Could you check a few things on this model? Use its own coordinates, in mm. Face numbers are marked on the shaded views. A direction names the side the tool comes from. Give positions to 0.01 mm unless a question says otherwise; leave off trailing zeros. Loops run counter-clockwise (first coordinate to the right, second up) from the corner with the lowest first, then second, coordinate; pieces in that order, holes last. Notation, with made-up numbers: (85, 57) - (142, 57) arc R28 ccw to (142, 81) - close; hole circle Ø4 at (34, 17). An arc over 180 degrees is marked (long way). Answer in a Markdown table with one row per item. Add a question column.
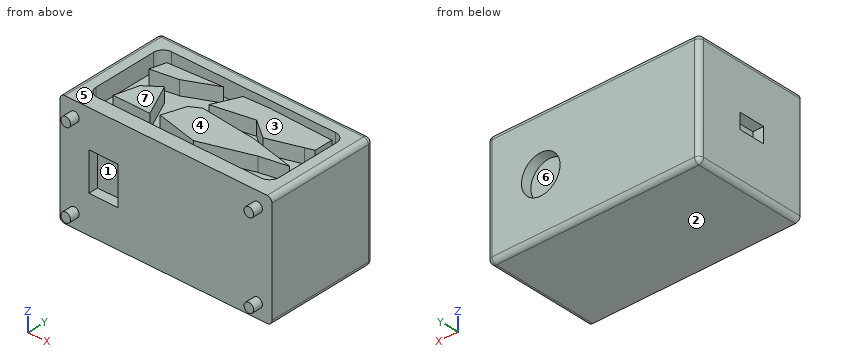
```python
from build123d import *

# Parameters (mm, degrees)
SKETCH1_W           = 220
SKETCH1_H           = 100
SKETCH1_W_2         = 184
SKETCH1_H_2         = 64
BOSS_EXTRUDE1_DEPTH = 80
SKETCH11_W          = 220
SKETCH11_H          = 100
BOSS_EXTRUDE6_DEPTH = 18
SKETCH12_W          = 220
SKETCH12_H          = 100
BOSS_EXTRUDE7_DEPTH = 18
SKETCH2_W           = 220
SKETCH2_H           = 116
SKETCH2_W_2         = 190
SKETCH2_H_2         = 86
BOSS_EXTRUDE2_DEPTH = 18
BOSS_EXTRUDE3_DEPTH = 15
FILLET9_R           = 5
FILLET8_R           = 10
SKETCH13_R          = 5
BOSS_EXTRUDE8_DEPTH = 10
SKETCH14_W          = 16
SKETCH14_H          = 27
CUT_EXTRUDE1_DEPTH  = 10
CUT_EXTRUDE1_DRAFT  = -6
SKETCH15_R          = 20
CUT_EXTRUDE2_DEPTH  = 10
CUT_EXTRUDE2_DRAFT  = -4
SKETCH17_W          = 30
SKETCH17_H          = 40
CUT_EXTRUDE3_DEPTH  = 10


with BuildPart() as part:
    # Sketch1 → Boss-Extrude1 (new body)
    with BuildSketch(Plane(origin=(0, 0, 0), x_dir=(1, 0, 0), z_dir=(0, 1, 0))):
        with Locations((19.985024942, -17.460570406)):
            Rectangle(SKETCH1_W, SKETCH1_H)
        with Locations((19.985024942, -17.460570406)):
            Rectangle(SKETCH1_W_2, SKETCH1_H_2, mode=Mode.SUBTRACT)
    extrude(amount=BOSS_EXTRUDE1_DEPTH)

    # Sketch11 → Boss-Extrude6 (add)
    with BuildSketch(Plane(origin=(0, 80, 0), x_dir=(1, 0, 0), z_dir=(0, 1, 0))):
        with Locations((19.985024942, -17.460570406)):
            Rectangle(SKETCH11_W, SKETCH11_H)
    extrude(amount=BOSS_EXTRUDE6_DEPTH)

    # Sketch12 → Boss-Extrude7 (add)
    with BuildSketch(Plane.XZ):
        with Locations((19.985024942, 17.460570406)):
            Rectangle(SKETCH12_W, SKETCH12_H)
    extrude(amount=BOSS_EXTRUDE7_DEPTH)

    # Sketch2 → Boss-Extrude2 (add)
    with BuildSketch(Plane.XY.offset(67.460570406)):
        with Locations((19.985024942, 40)):
            Rectangle(SKETCH2_W, SKETCH2_H)
        with Locations((19.985024942, 40)):
            Rectangle(SKETCH2_W_2, SKETCH2_H_2, mode=Mode.SUBTRACT)
    extrude(amount=BOSS_EXTRUDE2_DEPTH)

    # Sketch3 → Boss-Extrude3 (add)
    with BuildSketch(Plane.XY.offset(67.460570406)):
        Polygon((14.957915815, 76.501183659), (2.936567903, 50.272788216), (44.902000614, 58.797016735), (65.229007083, 43.497119393), (98.451641312, 54.534902475), (106.944672327, 57.35660028), (106.944672327, 76.501183659), (41.011301547, 77.951227522), align=None)
        Polygon((-60.667291048, 72.566924343), (-65.038690289, 56.611317114), (-37.280305111, 61.419856279), (-5.369090654, 76.501183659), align=None)
        Polygon((-54.547332111, 34.535750949), (-39.247434769, 46.119958937), (-22.636117654, 10.711625088), (-60.667291048, 10.711625088), align=None)
        Polygon((-7.554790274, 37.377160456), (-15.111155502, 14.241854245), (27.984608681, 4.591666151), (79.685296007, 21.768539242), (107.463223985, 27.410930863), (60.959158385, 37.824320409), (2.936567903, 43.497119393), align=None)
    extrude(amount=BOSS_EXTRUDE3_DEPTH)

    # Fillet9
    fillet9_edges = [part.edges().sort_by_distance(p)[0] for p in [
        (-90.014975058, 98, 26.460570406),
        (129.985024942, 98, 26.460570406),
        (19.985024942, 98, -32.539429594),
        (19.985024942, 98, 85.460570406),
        (-90.014975058, 40, 85.460570406),
        (129.985024942, 40, 85.460570406),
        (-90.014975058, 40, -32.539429594),
        (129.985024942, 40, -32.539429594),
    ]]
    fillet(fillet9_edges, radius=FILLET9_R)

    # Fillet8
    fillet8_edges = [part.edges().sort_by_distance(p)[0] for p in [
        (-75.014975058, 83, 76.460570406),
        (114.985024942, 83, 76.460570406),
        (114.985024942, -3, 76.460570406),
        (-75.014975058, -3, 76.460570406),
    ]]
    fillet(fillet8_edges, radius=FILLET8_R)

    # Sketch13 → Boss-Extrude8 (add)
    with BuildSketch(Plane.XZ.offset(18)):
        with Locations(Location((-75.014975058, 70.460570406, 0), (0, 0, 270))):
            Circle(SKETCH13_R)
        with Locations(Location((114.985024942, 70.460570406, 0), (0, 0, 90))):
            Circle(SKETCH13_R)
        with Locations(Location((114.985024942, -17.539429594, 0), (0, 0, 270))):
            Circle(SKETCH13_R)
        with Locations(Location((-75.014975058, -17.539429594, 0), (0, 0, 90))):
            Circle(SKETCH13_R)
    extrude(amount=BOSS_EXTRUDE8_DEPTH)


with BuildPart() as cut_extrude1_tool:
    # Sketch14 → Cut-Extrude1 (with draft: the straight prism first)
    with BuildSketch(Plane.ZY.offset(90.014975058)):
        with Locations((26.460570406, 37.5)):
            Rectangle(SKETCH14_W, SKETCH14_H)
    extrude(amount=-CUT_EXTRUDE1_DEPTH)
    # Cut-Extrude1: the draft: its side faces are tilted about the plane it starts from
    cut_extrude1_sides = [cut_extrude1_tool.faces().sort_by_distance(p)[0] for p in [
        (-85.014975058, 37.5, 18.460570406),
        (-85.014975058, 24, 26.460570406),
        (-85.014975058, 37.5, 34.460570406),
        (-85.014975058, 51, 26.460570406),
    ]]
    draft(cut_extrude1_sides, Plane.ZY.offset(90.014975058), CUT_EXTRUDE1_DRAFT)


with BuildPart() as part_1:
    add(part.part)

    # Cut-Extrude1: cut by cut_extrude1_tool
    add(cut_extrude1_tool.part, mode=Mode.SUBTRACT)


with BuildPart() as cut_extrude2_tool:
    # Sketch15 → Cut-Extrude2 (with draft: the straight prism first)
    with BuildSketch(Plane(origin=(0, 98, 0), x_dir=(1, 0, 0), z_dir=(0, 1, 0))):
        with Locations((74.457875253, -26.460570406)):
            Circle(SKETCH15_R)
    extrude(amount=-CUT_EXTRUDE2_DEPTH)
    # Cut-Extrude2: the draft: its side faces are tilted about the plane it starts from
    cut_extrude2_sides = [cut_extrude2_tool.faces().sort_by_distance(p)[0] for p in [
        (54.457875253, 93, 26.460570406),
    ]]
    draft(cut_extrude2_sides, Plane(origin=(0, 98, 0), x_dir=(1, 0, 0), z_dir=(0, 1, 0)), CUT_EXTRUDE2_DRAFT)


with BuildPart() as part_2:
    add(part_1.part)

    # Cut-Extrude2: cut by cut_extrude2_tool
    add(cut_extrude2_tool.part, mode=Mode.SUBTRACT)

    # Sketch17 → Cut-Extrude3 (cut)
    with BuildSketch(Plane.XZ.offset(18)):
        with Locations((-45.014975058, 26.460570406)):
            Rectangle(SKETCH17_W, SKETCH17_H)
    extrude(amount=-CUT_EXTRUDE3_DEPTH, mode=Mode.SUBTRACT)


solid = part_2.part
```
(1) I want a section at A-A on z = -5. Please give me the cut outline in (x, y).
(2) On a 3-axis mill with a long thin cutter (end or side, diameter ignored), from which of +Z, -Z, +X, -X, +Y, -Y can I reach the whole of each face in a straight line? I mean the marked faces 1, 2 and 3. Say none if no direction works.
(3) We'd pull the mould along Y, two halves only. Please class the marked faces 4, 5, 6 and 7: pulls with the +Y half, pulls with the -Y half, needs draft (parallel to the pull), parting line crosses it, or undercut.
(4) I want a section at D-D on y = 65.5. Please give me the cut outline in (x, z), then the cut area to 3 significant figures.
(5) For pin 1 Ø1 at (x, z) = (-28.5, 40.5) entering from -Y; pin 2 Ø10 at (x, y) = (81.5, 19) entering from +Z; pin 3 Ø10 at (x, z) = (-43.5, 23) entering from -Y, each with a flat end and sliding along its axis, tell me the tip position at first contact or that it passes through.
(6) I want a section at B-B on x = -25.5. Please give me the cut outline in (y, z), then the cut area to 3 significant figures.
(7) I want a section at C-C on y = 32. Please give me the cut outline in (x, z).
(8) Please list where these lines run through material, in increasing order: line 1 (Z direction, x = 102.5, y = 31); line 2 (X direction, y = 58.5, z = 17); line 3 (Y direction, x = 85, z = 68.5).
Reported:
| question | item | result |
|---|---|---|
| 1 | outline | (-90.01, -18) - (129.99, -18) - (129.99, 93) arc R5 ccw to (124.99, 98) - (-85.01, 98) arc R5 ccw to (-90.01, 93) - close; hole (-72.01, 0) - (111.99, 0) - (111.99, 80) - (-72.01, 80) - close |
| 2 | face 1 | -Y |
| 2 | face 2 | -Z, +X, -X, +Y, -Y |
| 2 | face 3 | +Z |
| 3 | face 4 | undercut |
| 3 | face 5 | needs draft |
| 3 | face 6 | pulls with the +Y half |
| 3 | face 7 | undercut |
| 4 | outline | (-90.01, -27.54) arc R5 ccw to (-85.01, -32.54) - (124.99, -32.54) arc R5 ccw to (129.99, -27.54) - (129.99, 80.46) arc R5 ccw to (124.99, 85.46) - (114.99, 85.46) - (114.99, 67.46) - (106.94, 67.46) - (106.94, 82.46) - (9.92, 82.46) - (9.92, 67.46) - (-28.65, 67.46) - (-28.65, 82.46) - (-62.6, 82.46) - (-62.6, 67.46) - (-75.01, 67.46) - (-75.01, 85.46) - (-85.01, 85.46) arc R5 ccw to (-90.01, 80.46) - close; hole (-72.01, -14.54) - (111.99, -14.54) - (111.99, 49.46) - (-72.01, 49.46) - close |
| 4 | area | 12,700 mm² |
| 5 | pin 1 | y = -18 |
| 5 | pin 2 | z = 82.46 |
| 5 | pin 3 | y = -8 |
| 6 | outline | (-18, -32.54) - (93, -32.54) arc R5 ccw to (98, -27.54) - (98, 80.46) arc R5 ccw to (93, 85.46) - (83, 85.46) - (83, 67.46) - (75.07, 67.46) - (75.07, 82.46) - (66.99, 82.46) - (66.99, 67.46) - (16.82, 67.46) - (16.82, 82.46) - (10.71, 82.46) - (10.71, 67.46) - (-3, 67.46) - (-3, 85.46) - (-18, 85.46) - close; hole (0, -14.54) - (80, -14.54) - (80, 49.46) - (0, 49.46) - close |
| 6 | area | 7,220 mm² |
| 7 | outline | (-90.01, -27.54) arc R5 ccw to (-85.01, -32.54) - (124.99, -32.54) arc R5 ccw to (129.99, -27.54) - (129.99, 80.46) arc R5 ccw to (124.99, 85.46) - (114.99, 85.46) - (114.99, 67.46) - (86.97, 67.46) - (86.97, 82.46) - (-9.31, 82.46) - (-9.31, 67.46) - (-32.62, 67.46) - (-32.62, 82.46) - (-55.2, 82.46) - (-55.2, 67.46) - (-75.01, 67.46) - (-75.01, 85.46) - (-85.01, 85.46) arc R5 ccw to (-90.01, 80.46) - (-90.01, 34.46) - (-80.01, 33.41) - (-80.01, 19.51) - (-90.01, 18.46) - close; hole (-72.01, -14.54) - (111.99, -14.54) - (111.99, 49.46) - (-72.01, 49.46) - close |
| 8 | line 1 | -32.54 to -14.54, 49.46 to 67.46 |
| 8 | line 2 | -90.01 to -72.01, 111.99 to 129.99 |
| 8 | line 3 | -18 to -3, 22.85 to 32.44, 50.07 to 76.98, 83 to 98 |
